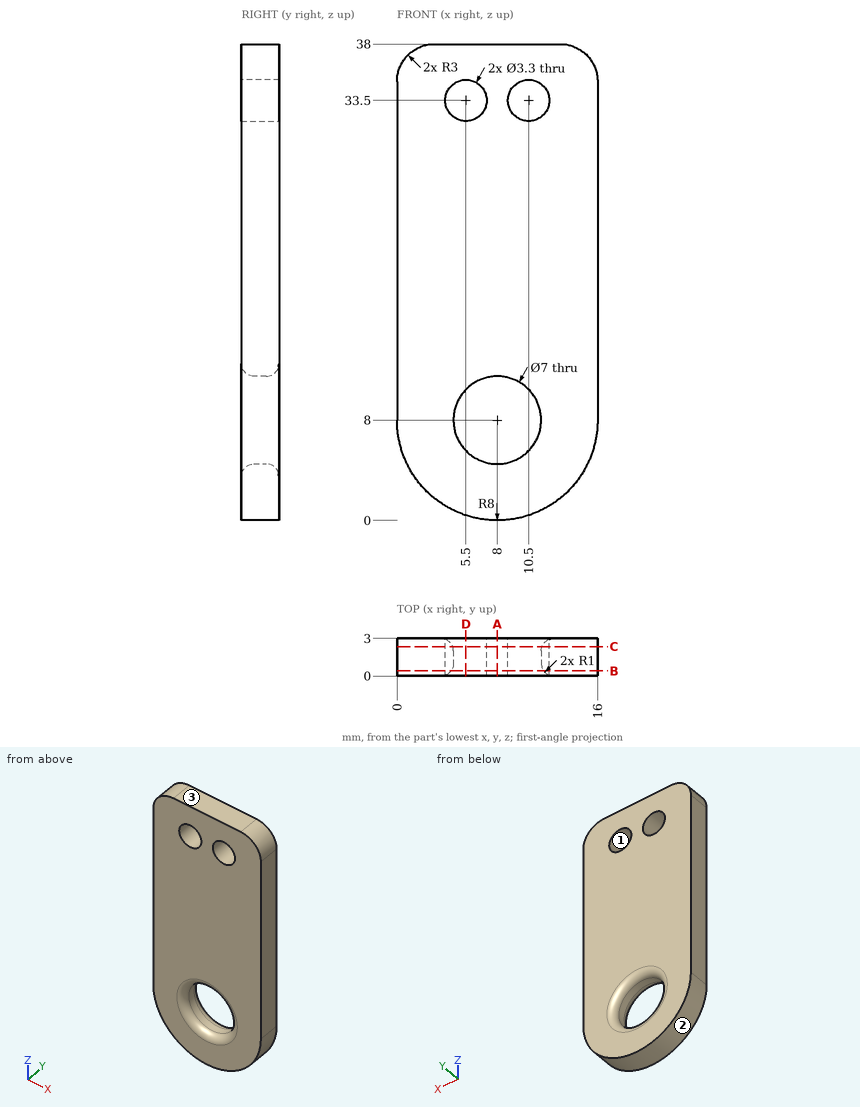
Check sheet for the drawn part. Datum: minimum x, y, z corner. Units: mm. Round coordinates to 2 decimals unless told otherwise and drop trailing zeros. Order: outer loops, then holes, each group sorted by start corner. A loop starts at its lowest first (then second) coordinate and runs counter-clockwise, first axis right, second up. Notation, with made-up numbers: (49, 32.25) -> (67, 32.25) arc R17 ccw to (67, 65.25) -> close; hole circle Ø2 at (57, 82). An arc over 180 degrees is marked (long way). Put each result on its own line as item: value. Start each with the question number.
(1) Draft check along Z on the marked faces 1, 2 and 3. Enter one of: +Z half, -Z half, draft (parallel to the pull), parting line (faces both ways), or undercut.
(2) Depth check by flat-ended pin: pin 1 Ø5 at (x, z) = (9, 7) entering from -Y; pin 2 Ø3 at (x, z) = (10.5, 33.5) entering from -Y; pin 3 Ø8 at (x, z) = (8, 8) entering from +Y. Enter the tip coordinate at first touch or a pass-through.
(3) Section check C-C (y = 2.35). Enter the section's corners in (x, z).
(4) Section check B-B (y = 0.4). Enter the section's corners in (x, z).
(5) Section check D-D (x = 5.5). State how many separate pieces and enclosed holes the cut face has, then the cut area to 3 significant figures.
(6) Section check A-A (x = 8). Enter the section's corners in (y, z), then the cut area to 3 significant figures.
(7) Material ranges on line 1 along X through (y, z) = (1.4, 8); line 2 along X through (y, z) = (1.85, 34.5); line 3 along Z through (x, y) = (9.5, 1.4), recorded low to high.
Completed:
1. face 1: undercut
1. face 2: -Z half
1. face 3: +Z half
2. pin 1: stops at y = 0.19
2. pin 2: passes through
2. pin 3: stops at y = 2.87
3. outline: (0, 8) arc R8 ccw to (16, 8) -> (16, 35) arc R3 ccw to (13, 38) -> (3, 38) arc R3 ccw to (0, 35) -> close; hole circle Ø3.3 at (5.5, 33.5); hole circle Ø7.13 at (8, 8); hole circle Ø3.3 at (10.5, 33.5)
4. outline: (0, 8) arc R8 ccw to (16, 8) -> (16, 35) arc R3 ccw to (13, 38) -> (3, 38) arc R3 ccw to (0, 35) -> close; hole circle Ø3.3 at (5.5, 33.5); hole circle Ø7.4 at (8, 8); hole circle Ø3.3 at (10.5, 33.5)
5. separate pieces: 3
5. enclosed holes: 0
5. area: 87.0 mm2
6. outline: (0, 0) -> (3, 0) -> (3, 3.5) arc R1 ccw to (2, 4.5) -> (1, 4.5) arc R1 ccw to (0, 3.5) -> close; (0, 12.5) arc R1 ccw to (1, 11.5) -> (2, 11.5) arc R1 ccw to (3, 12.5) -> (3, 38) -> (0, 38) -> close
6. area: 92.1 mm2
7. line 1: x = 0 to 4.5, 11.5 to 16
7. line 2: x = 0 to 4.19, 6.81 to 9.19, 11.81 to 16
7. line 3: z = 0.14 to 4.84, 11.16 to 32.19, 34.81 to 38
